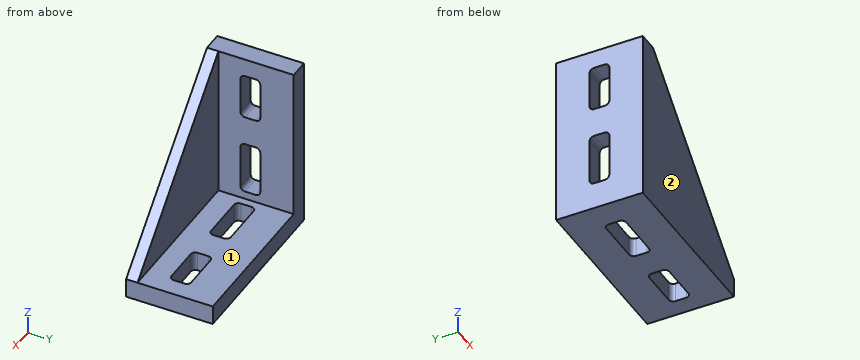
from build123d import *

# Parameters (mm, degrees)
F0_W     = 76
F0_H     = 38
F1_DEPTH = 76
F3_DEPTH = 38.001
F4_DEPTH = 33
F6_DEPTH = 76.001
F8_DEPTH = 76.001


with BuildPart() as f1:
    # F0 (on Top) → F1 (new body)
    with BuildSketch(Plane.XY):
        Rectangle(F0_W, F0_H)
    extrude(amount=F1_DEPTH)

    # F2 (on face) → F3 (cut, through all)
    with BuildSketch(Plane(origin=(0, 19, 0), x_dir=(-1, 0, 0), z_dir=(0, 1, 0))):
        Polygon((-38, 8.5), (29.5, 76), (-38, 76), align=None)
    extrude(amount=-F3_DEPTH, mode=Mode.SUBTRACT)

    # F2 (on face) → F4 (cut)
    with BuildSketch(Plane(origin=(0, 19, 0), x_dir=(-1, 0, 0), z_dir=(0, 1, 0))):
        Polygon((29.5, 8.5), (29.5, 76), (-38, 8.5), align=None)
    extrude(amount=-F4_DEPTH, mode=Mode.SUBTRACT)

    # F5 (on face) → F6 (cut, through all)
    with BuildSketch(Plane(origin=(-38, 0, 0), x_dir=(0, -1, 0), z_dir=(-1, 0, 0))):
        with BuildLine():
            Line((2.35, 68), (-2.35, 68))
            ThreePointArc((-2.35, 68), (-3.764214, 67.414214), (-4.35, 66))
            Line((-4.35, 66), (-4.35, 50))
            ThreePointArc((-4.35, 50), (-3.764214, 48.585786), (-2.35, 48))
            Line((-2.35, 48), (2.35, 48))
            ThreePointArc((2.35, 48), (3.764214, 48.585786), (4.35, 50))
            Line((4.35, 50), (4.35, 66))
            ThreePointArc((4.35, 66), (3.764214, 67.414214), (2.35, 68))
        make_face()
        with BuildLine():
            Line((2.35, 35), (-2.35, 35))
            ThreePointArc((-2.35, 35), (-3.764214, 34.414214), (-4.35, 33))
            Line((-4.35, 33), (-4.35, 14))
            ThreePointArc((-4.35, 14), (-3.764214, 12.585786), (-2.35, 12))
            Line((-2.35, 12), (2.35, 12))
            ThreePointArc((2.35, 12), (3.764214, 12.585786), (4.35, 14))
            Line((4.35, 14), (4.35, 33))
            ThreePointArc((4.35, 33), (3.764214, 34.414214), (2.35, 35))
        make_face()
    extrude(amount=-F6_DEPTH, mode=Mode.SUBTRACT)

    # F7 (on face) → F8 (cut, through all)
    with BuildSketch(Plane(origin=(0, 0, 0), x_dir=(1, 0, 0), z_dir=(0, 0, -1))):
        with BuildLine():
            Line((-3, -2.35), (-3, 2.35))
            ThreePointArc((-3, 2.35), (-3.585786, 3.764214), (-5, 4.35))
            Line((-5, 4.35), (-24, 4.35))
            ThreePointArc((-24, 4.35), (-25.414214, 3.764214), (-26, 2.35))
            Line((-26, 2.35), (-26, -2.35))
            ThreePointArc((-26, -2.35), (-25.414214, -3.764214), (-24, -4.35))
            Line((-24, -4.35), (-5, -4.35))
            ThreePointArc((-5, -4.35), (-3.585786, -3.764214), (-3, -2.35))
        make_face()
        with BuildLine():
            Line((30, -2.35), (30, 2.35))
            ThreePointArc((30, 2.35), (29.414214, 3.764214), (28, 4.35))
            Line((28, 4.35), (12, 4.35))
            ThreePointArc((12, 4.35), (10.585786, 3.764214), (10, 2.35))
            Line((10, 2.35), (10, -2.35))
            ThreePointArc((10, -2.35), (10.585786, -3.764214), (12, -4.35))
            Line((12, -4.35), (28, -4.35))
            ThreePointArc((28, -4.35), (29.414214, -3.764214), (30, -2.35))
        make_face()
    extrude(amount=-F8_DEPTH, mode=Mode.SUBTRACT)


solid = f1.part
For this review, take the finished solid that the model builds, in its own axes (mm). Face numbers are marked on the shaded views. A direction names the side the tool comes from. Coordinates: 2 decimals unless noted, no trailing zeros. Write each loop counter-clockwise with the first axis right and the second up, starting at its lowest first coordinate (ties: lowest second). Pieces come first, ordered by that corner, then holes. Notation, with made-up numbers: (-5, 7.25) -> (15, 7.25) arc R26 ccw to (15, 40.25) -> close; hole circle Ø3 at (-20.75, 31). An arc over 180 degrees is marked (long way). Write each question's results on one line, items separated by ' | '. Start each with the question number.
1) Consider section D-D (z = 37). Write out the cut boundary in (x, y).
2) Consider section B-B (z = 28). Write out the cut boundary in (x, y).
3) Consider section C-C (x = 32). Write out the cut boundary in (y, z).
4) Consider section A-A (x = -16). Write out the cut boundary in (y, z).
5) Wall thickness on L1, parallel to Y at x = -33.5, z = 55; L2, parallel to X at y = 16, z = 59.5; L3, parallel to Y at x = 22, z = 14: over which ranges is each line inside the solid? List them lowest first. Write a range as [from, to].
6) For the marked faces 1 and 2, list the 3-axis set-ups (+Z, -Z, +X, -X, +Y, -Y) from which the entire face can be reached by the end or side of a thin tool; tool diameter is ignored.
7) Insertion check: pin 1 (16.5 mm diameter, centred on x = 16, y = 7.5, fed in from +Z); pin 2 (10 mm diameter, centred on y = -1.5, z = 49.5, fed in from +X); pin 3 (4 mm diameter, centred on x = 24, y = 2, fed in from +Z); pin 4 (8 mm diameter, centred on x = 22, z = 28, fed in from +Y). Each pin has a flat end and moves straight along its axis. Give the tip position at first contact, or say it passes through.
Geometry says:
1) outline: (-38, -19) -> (9.5, -19) -> (9.5, -14) -> (-29.5, -14) -> (-29.5, 19) -> (-38, 19) -> close
2) outline: (-38, -19) -> (18.5, -19) -> (18.5, -14) -> (-29.5, -14) -> (-29.5, -4.35) -> (-38, -4.35) -> close; (-38, 4.35) -> (-29.5, 4.35) -> (-29.5, 19) -> (-38, 19) -> close
3) outline: (-19, 0) -> (19, 0) -> (19, 8.5) -> (-14, 8.5) -> (-14, 14.5) -> (-19, 14.5) -> close
4) outline: (-19, 0) -> (-4.35, 0) -> (-4.35, 8.5) -> (-14, 8.5) -> (-14, 62.5) -> (-19, 62.5) -> close; (4.35, 0) -> (19, 0) -> (19, 8.5) -> (4.35, 8.5) -> close
5) L1: [-19, -4.35], [4.35, 19] | L2: [-38, -29.5] | L3: [-19, -14]
6) face 1: +Z, +X, +Y | face 2: +Z, -Z, +X, -X, -Y
7) pin 1: z = 8.5 | pin 2: x = -29.5 | pin 3: through | pin 4: y = -14
